Geometry: see drawing. Coordinates: mm, zero at the bounding-box minimum. A direction names the side the tool comes from. Coordinates: 2 decimals unless noted, no trailing zeros. Order: outer loops, then holes, each group sorted by start corner. A loop starts at its lowest first (then second) coordinate and runs counter-clockwise, first axis right, second up. Notation, with made-up numbers: M 5.5,42.5 L 54.5,42.5 A25 ccw 54.5,59.5 Z; hole C -39,-15 d4. An arc over 180 degrees is marked long. Answer in a Markdown table with one row per item.
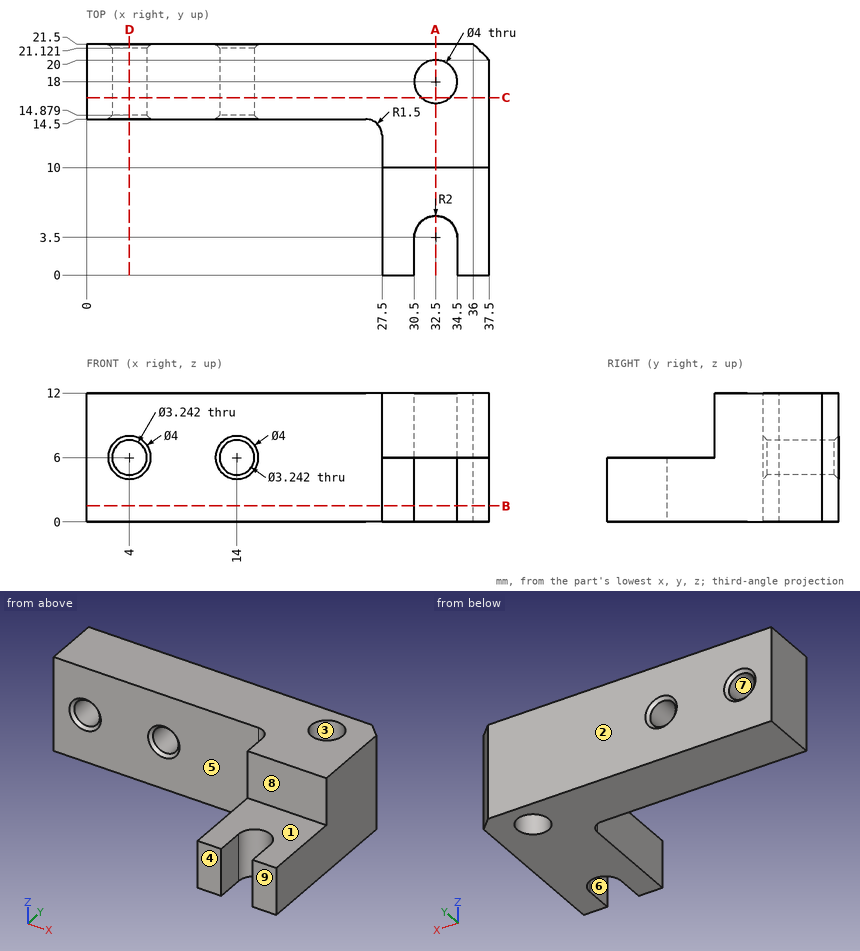
1) Mould query, pull axis Y, two halves, no side actions, for the marked faces 1, 2, 3 and 4. Classes: +Y half, -Y half, draft (parallel to the pull), parting line (faces both ways), or undercut.
Resolved:
| item | result |
|---|---|
| face 1 | draft |
| face 2 | +Y half |
| face 3 | undercut |
| face 4 | -Y half |
2) Contact query for flat-ended pins moving along their axis: pin 1 (5 mm diameter, centred on x = 32.5, y = 3, fed in from +Z); pin 2 (1.5 mm diameter, centred on x = 25, z = 2, fed in from -Y); pin 3 (3 mm diameter, centred on x = 30, z = 9, fed in from -Y). Output: stop coordinate, or through.
Resolved:
| item | result |
|---|---|
| pin 1 | stops at z = 6 |
| pin 2 | stops at y = 14.5 |
| pin 3 | stops at y = 10 |
3) Cut plane B-B, the plane z = 1.5. Output: boundary loops of the cut face in (x, y), and give its area (3 significant figures).
Resolved:
| item | result |
|---|---|
| outline | M 0,14.5 L 26,14.5 A1.5 cw 27.5,13 L 27.5,0 L 30.5,0 L 30.5,3.5 A2 cw 34.5,3.5 L 34.5,0 L 37.5,0 L 37.5,20 L 36,21.5 L 0,21.5 Z; hole C 32.5,18 d4 |
| area | 374 mm2 |
4) Cut plane D-D, the plane x = 4. Output: boundary loops of the cut face in (y, z).
Resolved:
| item | result |
|---|---|
| outline | M 14.5,0 L 21.5,0 L 21.5,4 L 21.12,4.38 L 14.88,4.38 L 14.5,4 Z; M 14.5,8 L 14.88,7.62 L 21.12,7.62 L 21.5,8 L 21.5,12 L 14.5,12 Z |
5) Reachability of the marked faces 5, 6, 7, 8 and 9 from +Z, -Z, +X, -X, +Y, -Y: full face, straight path, thin tool, end or side. Return the list, or none.
Resolved:
| item | result |
|---|---|
| face 5 | +Z, -Z, -X, -Y |
| face 6 | +Z, -Z, -Y |
| face 7 | +Y, -Y |
| face 8 | +Z, +X, -X, -Y |
| face 9 | +Z, -Z, +X, -X, -Y |
6) Cut plane A-A, the plane x = 32.5. Output: boundary loops of the cut face in (y, z), and give its area (3 significant figures).
Resolved:
| item | result |
|---|---|
| outline | M 5.5,0 L 16,0 L 16,12 L 10,12 L 10,6 L 5.5,6 Z; M 20,0 L 21.5,0 L 21.5,12 L 20,12 Z |
| area | 117 mm2 |
7) Cut plane C-C, the plane y = 16.5. Output: boundary loops of the cut face in (x, z), and give its area (3 significant figures).
Resolved:
| item | result |
|---|---|
| outline | M 0,0 L 31.18,0 L 31.18,12 L 0,12 Z; M 33.82,0 L 37.5,0 L 37.5,12 L 33.82,12 Z; hole C 4,6 d3.24; hole C 14,6 d3.24 |
| area | 402 mm2 |
8) Material intervals for probe 1 along X at (y, z) = (18, 5.5); probe 2 along Y at (x, z) = (22.5, 11.75); probe 3 along X at (y, z) = (18, 3.25), sorted ascending.
Resolved:
| item | result |
|---|---|
| probe 1 | x = 0 to 2.46, 5.54 to 12.46, 15.54 to 30.5, 34.5 to 37.5 |
| probe 2 | y = 14.5 to 21.5 |
| probe 3 | x = 0 to 30.5, 34.5 to 37.5 |
